from build123d import *

# Parameters (mm, degrees)
SKETCH_1_R          = 1.5
EXTRUDE_1_DEPTH     = 1.5
SKETCH_2_R          = 1.5
SKETCH_2_R_2        = 8.3
CUT_EXTRUDE_1_DEPTH = 10


with BuildPart() as part:
    # 草图1 → 凸台-拉伸1 (new body)
    with BuildSketch(Plane.XY):
        Polygon((-44, -22), (-20.444109017, -35.6), (20.444109017, -35.6), (44, -22), (44, 22), (38, 28), (-38, 28), (-44, 22), align=None)
        with Locations((-41, 19)):
            Circle(SKETCH_1_R, mode=Mode.SUBTRACT)
        with Locations((-41, -19)):
            Circle(SKETCH_1_R, mode=Mode.SUBTRACT)
        with Locations((41, 19)):
            Circle(SKETCH_1_R, mode=Mode.SUBTRACT)
        with Locations((41, -19)):
            Circle(SKETCH_1_R, mode=Mode.SUBTRACT)
    extrude(amount=EXTRUDE_1_DEPTH)

    # 草图2 → 切除-拉伸1 (cut)
    with BuildSketch(Plane.XY.offset(1.5)):
        with Locations((0, -0.2)):
            Circle(SKETCH_2_R)
        with Locations((-18.8, -19)):
            Circle(SKETCH_2_R)
        with Locations((18.8, -19)):
            Circle(SKETCH_2_R)
        with Locations((0, -19)):
            Circle(SKETCH_2_R_2)
        with Locations((-15.444109017, -32.6)):
            Circle(SKETCH_2_R)
        with Locations((15.444109017, -32.6)):
            Circle(SKETCH_2_R)
        with Locations((-35, 25)):
            Circle(SKETCH_2_R)
        with Locations((35, 25)):
            Circle(SKETCH_2_R)
    extrude(amount=-CUT_EXTRUDE_1_DEPTH, mode=Mode.SUBTRACT)


solid = part.part
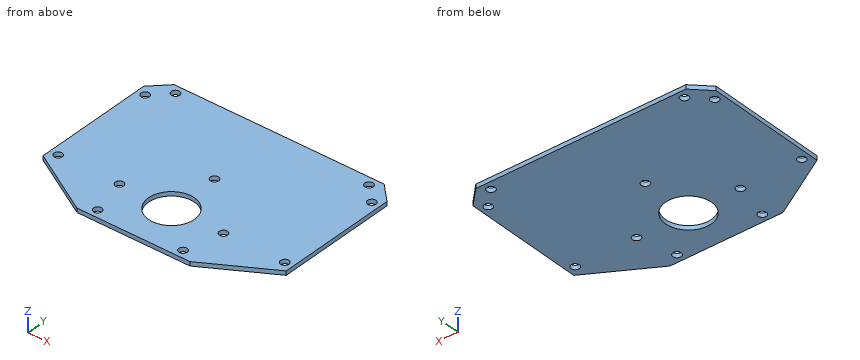
Here's how the part is built. I have some questions about the finished solid (model axes, mm). Coordinates: 2 decimals unless noted, no trailing zeros. Loops run counter-clockwise (first coordinate to the right, second up) from the corner with the lowest first, then second, coordinate; pieces in that order, holes last.
1. Imagine slicing it at D-D, the plane y = -19. Please give me the cut outline in (x, z).
2. Imagine slicing it at A-A, the plane x = -18.8. Please give me the cut outline in (y, z).
3. Imagine slicing it at B-B, the plane y = 25. Please give me the cut outline in (x, z), and give its area (3 significant figures).
4. Imagine slicing it at C-C, the plane x = 0. Please give me the cut outline in (y, z).
5. I need wall thicknesses on L1, parallel to Y at x = 0, z = 0.6; L2, parallel to Y at x = 18.8, z = 1.15; L3, parallel to X at y = -21, z = 1. Which ranges of each line are inside material? Lowest first, please.
Taken from the geometry:
1. outline: (-44, 0) - (-42.5, 0) - (-42.5, 1.5) - (-44, 1.5) - close; (-39.5, 0) - (-20.3, 0) - (-20.3, 1.5) - (-39.5, 1.5) - close; (-17.3, 0) - (-8.3, 0) - (-8.3, 1.5) - (-17.3, 1.5) - close; (8.3, 0) - (17.3, 0) - (17.3, 1.5) - (8.3, 1.5) - close; (20.3, 0) - (39.5, 0) - (39.5, 1.5) - (20.3, 1.5) - close; (42.5, 0) - (44, 0) - (44, 1.5) - (42.5, 1.5) - close
2. outline: (-35.6, 0) - (-20.5, 0) - (-20.5, 1.5) - (-35.6, 1.5) - close; (-17.5, 0) - (28, 0) - (28, 1.5) - (-17.5, 1.5) - close
3. outline: (-41, 0) - (-36.5, 0) - (-36.5, 1.5) - (-41, 1.5) - close; (-33.5, 0) - (33.5, 0) - (33.5, 1.5) - (-33.5, 1.5) - close; (36.5, 0) - (41, 0) - (41, 1.5) - (36.5, 1.5) - close
3. area: 114 mm2
4. outline: (-35.6, 0) - (-27.3, 0) - (-27.3, 1.5) - (-35.6, 1.5) - close; (-10.7, 0) - (-1.7, 0) - (-1.7, 1.5) - (-10.7, 1.5) - close; (1.3, 0) - (28, 0) - (28, 1.5) - (1.3, 1.5) - close
5. L1: y = -35.6 to -27.3, -10.7 to -1.7, 1.3 to 28
5. L2: y = -35.6 to -20.5, -17.5 to 28
5. L3: x = -44 to -8.06, 8.06 to 44
